```python
from build123d import *

# Parameters (mm, degrees)
F1_DEPTH = 70
F3_DEPTH = 75.001
F5_DEPTH = 66.001


with BuildPart() as f1:
    # F0 (on Right) → F1 (new body, symmetric)
    with BuildSketch(Plane.YZ):
        Polygon((-37.5, -33), (37.5, -33), (37.5, 33), (0, 13), (-37.5, 33), align=None)
    extrude(amount=F1_DEPTH, both=True)

    # F2 (on face) → F3 (cut, through all)
    with BuildSketch(Plane.XZ.offset(37.5)):
        Polygon((10, -13), (40, -13), (70, -33), (70, 33), (10, 33), align=None)
    extrude(amount=-F3_DEPTH, mode=Mode.SUBTRACT)

    # F4 (on face) → F5 (cut, through all)
    with BuildSketch(Plane(origin=(0, 0, -33), x_dir=(1, 0, 0), z_dir=(0, 0, -1))):
        Polygon((-70, -37.5), (-40, 0), (-70, 37.5), align=None)
    extrude(amount=-F5_DEPTH, mode=Mode.SUBTRACT)


solid = f1.part
```
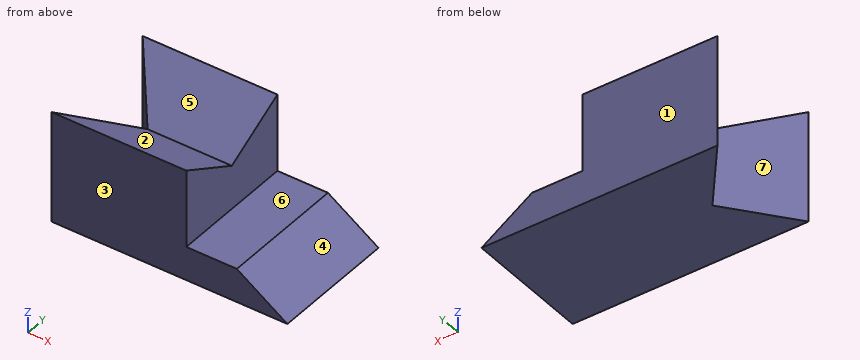
Part model, mm, in its own coordinate system. Face numbers are marked on the shaded views. A direction names the side the tool comes from. Round coordinates to 2 decimals unless told otherwise and drop trailing zeros. Write each loop counter-clockwise with the first axis right and the second up, starting at its lowest first coordinate (ties: lowest second). Pieces come first, ordered by that corner, then holes. Notation, with made-up numbers: (48, 19) -> (76, 19) arc R23 cw to (76, 49) -> close; hole circle Ø9 at (63, 51). An arc over 180 degrees is marked (long way). Return JSON: item names as keys, results as strings. Group by question number.
Q1. Saw through at A-A on z = 21. Write the cut outline in (x, y), plus the area to 4 significant figures.
Q2. Probe L1, parallel to Y at x = -2, z = 18.5; L2, parallel to Y at x = -37.5, z = 29.5; L3, parallel to Z at x = 10.5, y = -28. List the from-to ranges inside material, lowest first. Write a range as [from, to].
Q3. Saw through at D-D on z = -21. Write the cut outline in (x, y).
Q4. Saw through at B-B on y = 16.5. Write the cut outline in (x, z), plus the area to 3 significant figures.
Q5. Saw through at C-C on x = -38.5. Write the cut outline in (y, z).
Q6. Pin check, flat tips, straight feed: pin 1 (10 mm diameter, centred on y = 13.5, z = 9, fed in from -X); pin 2 (12 mm diameter, centred on y = 21, z = -11, fed in from -X); pin 3 (6 mm diameter, centred on x = 51, y = -13.5, fed in from +Z). Stop position of each tip, or through.
Q7. Which spindle directions (+Z, -Z, +X, -X, +Y, -Y) get a long thin tool onto all of the face, cutting with end or side? Do the marked faces 5, 6 and 7. Say none if no direction does.
Q8. Mould opens along Y. For the marked faces 1, 2, 3 and 4 say: pulls with the +Y half, pulls with the -Y half, needs draft (parallel to the pull), parting line crosses it, or undercut.
Answer:
{
 "1": {"outline": "(-70, -37.5) -> (10, -37.5) -> (10, -15) -> (-52, -15) -> close; (-70, 37.5) -> (-52, 15) -> (10, 15) -> (10, 37.5) -> close", "area": "3,195 mm2"},
 "2": {"L1": "[-37.5, -10.31], [10.31, 37.5]", "L2": "[-37.5, -30.94], [30.94, 37.5]", "L3": "[-33, -13]"},
 "3": {"outline": "(-70, -37.5) -> (52, -37.5) -> (52, 37.5) -> (-70, 37.5) -> (-40, 0) -> close"},
 "4": {"outline": "(-53.2, -33) -> (70, -33) -> (40, -13) -> (10, -13) -> (10, 21.8) -> (-53.2, 21.8) -> close", "area": "4,360 mm2"},
 "5": {"outline": "(-37.5, -33) -> (37.5, -33) -> (37.5, 33) -> (0, 13) -> (-37.5, 33) -> close"},
 "6": {"pin 1": "x = -54.8", "pin 2": "x = -61.6", "pin 3": "z = -18.33"},
 "7": {"face 5": "+Z, +X, -X", "face 6": "+Z, +X, +Y, -Y", "face 7": "+Z, -Z, -X"},
 "8": {"face 1": "pulls with the +Y half", "face 2": "undercut", "face 3": "pulls with the -Y half", "face 4": "needs draft"}
}
